For this review, take the finished solid that the model builds, in its own axes (mm). A direction names the side the tool comes from. Round coordinates to 2 decimals unless told otherwise and drop trailing zeros. Loops run counter-clockwise (first coordinate to the right, second up) from the corner with the lowest first, then second, coordinate; pieces in that order, holes last.
1. Clearance check with flat-ended pins moving along their axes: pin 1 Ø1 at (y, z) = (14.5, -11.5) entering from -X; pin 2 Ø2.5 at (x, z) = (10, -6) entering from -Y; pin 3 Ø5 at (x, z) = (10, -20) entering from +Y. State where each tip first meets the part, or that it passes through.
2. Consider section C-C on y = 48. State the section outline as (x, z) points, then the cut area to 3 significant figures.
3. Consider section D-D on z = -13. State the section outline as (x, y) points, then the cut area to 3 significant figures.
4. Tool access review of faces 4 (the flat face through (0, 1, -13)), 5 (the flat face through (41, 27, -1)), 6 (the flat face through (42, 38, -23)): name each direction out of +Z, -Z, +X, -X, +Y, -Y from which nothing blocks a thin tool from reaching the whole face with its end or side.
5. Draft analysis for pull direction Y (two halves, no side actions). For faces 1 (the flat face through (22, 0, -13)), 2 (the flat face through (42, 23, -26)), 3 (the cylindrical face through (42.479, 60.336, -18.325)), state which applies: released by +Y, released by -Y, zero draft, split by the parting line, or undercut.
6. Consider section A-A on y = 14.5. State the section outline as (x, z) points, then the cut area to 3 significant figures.
7. To check wall thickness, follow line 1 along Y through (x, z) = (43.2, -8); line 2 along X through (y, z) = (1, -13); line 3 along Y through (x, z) = (4, -2.5). State the ranges of each line that lie inside material, in increasing order.
8. Consider section B-B on x = 3. State the section outline as (y, z) points, then the cut area to 3 significant figures.
from build123d import *

# Parameters (mm, degrees)
CROQUIS1_R              = 1.5
CROQUIS1_R_2            = 1.58
SALIENTE_EXTRUIR1_DEPTH = 3
CROQUIS2_W              = 3
CROQUIS2_H              = 26
SALIENTE_EXTRUIR2_DEPTH = 15
CROQUIS3_R              = 1.5
CORTAR_EXTRUIR1_DEPTH   = 15
CROQUIS4_W              = 3
CROQUIS4_H              = 3
SALIENTE_EXTRUIR3_DEPTH = 40.3
CROQUIS5_W              = 3
CROQUIS5_H              = 26
SALIENTE_EXTRUIR5_DEPTH = 7.5
CROQUIS6_R              = 1.5
CORTAR_EXTRUIR2_DEPTH   = 7.5


with BuildPart() as part:
    # Croquis1 → Saliente-Extruir1 (new body)
    with BuildSketch(Plane(origin=(0, 0, 0), x_dir=(1, 0, 0), z_dir=(0, 1, 0))):
        with BuildLine():
            Line((0, 1.5), (0, 24.5))
            ThreePointArc((0, 24.5), (0.439339828, 25.560660172), (1.5, 26))
            Line((1.5, 26), (44, 26))
            Line((44, 26), (44, 0))
            Line((44, 0), (1.5, 0))
            ThreePointArc((1.5, 0), (0.439339828, 0.439339828), (0, 1.5))
        make_face()
        with Locations(Location((10, 13, 0), (0, 0, 270))):
            Circle(CROQUIS1_R, mode=Mode.SUBTRACT)
        with Locations(Location((17, 13, 0), (0, 0, 270))):
            Circle(CROQUIS1_R, mode=Mode.SUBTRACT)
        with Locations(Location((10, 20, 0), (0, 0, 270))):
            Circle(CROQUIS1_R, mode=Mode.SUBTRACT)
        with Locations(Location((10, 6, 0), (0, 0, 270))):
            Circle(CROQUIS1_R, mode=Mode.SUBTRACT)
        with Locations(Location((3, 13, 0), (0, 0, 270))):
            Circle(CROQUIS1_R_2, mode=Mode.SUBTRACT)
    extrude(amount=SALIENTE_EXTRUIR1_DEPTH)

    # Croquis2 → Saliente-Extruir2 (add)
    with BuildSketch(Plane(origin=(0, 3, 0), x_dir=(1, 0, 0), z_dir=(0, 1, 0))):
        with Locations((42.5, 13)):
            Rectangle(CROQUIS2_W, CROQUIS2_H)
    extrude(amount=SALIENTE_EXTRUIR2_DEPTH)

    # Croquis3 → Cortar-Extruir1 (cut)
    with BuildSketch(Plane.ZY.offset(-41)):
        with Locations((-18, 14.5)):
            Circle(CROQUIS3_R)
        with Locations((-8, 14.5)):
            Circle(CROQUIS3_R)
    extrude(amount=-CORTAR_EXTRUIR1_DEPTH, mode=Mode.SUBTRACT)

    # Croquis4 → Saliente-Extruir3 (add)
    with BuildSketch(Plane(origin=(0, 18, 0), x_dir=(1, 0, 0), z_dir=(0, 1, 0))):
        with Locations((42.5, 24.5)):
            Rectangle(CROQUIS4_W, CROQUIS4_H)
        with Locations((42.5, 1.5)):
            Rectangle(CROQUIS4_W, CROQUIS4_H)
    extrude(amount=SALIENTE_EXTRUIR3_DEPTH)

    # Croquis5 → Saliente-Extruir5 (add)
    with BuildSketch(Plane(origin=(0, 58.3, 0), x_dir=(1, 0, 0), z_dir=(0, 1, 0))):
        with Locations((42.5, 13)):
            Rectangle(CROQUIS5_W, CROQUIS5_H)
    extrude(amount=SALIENTE_EXTRUIR5_DEPTH)

    # Croquis6 → Cortar-Extruir2 (cut)
    with BuildSketch(Plane.ZY.offset(-41)):
        with Locations((-18, 61.8)):
            Circle(CROQUIS6_R)
        with Locations((-8, 61.8)):
            Circle(CROQUIS6_R)
    extrude(amount=-CORTAR_EXTRUIR2_DEPTH, mode=Mode.SUBTRACT)


solid = part.part
Resolved:
1. pin 1: stops at x = 41
1. pin 2: passes through
1. pin 3: stops at y = 3
2. outline: (41, -26) - (44, -26) - (44, -23) - (41, -23) - close; (41, -3) - (44, -3) - (44, 0) - (41, 0) - close
2. area: 18.0 mm2
3. outline: (0, 0) - (1.42, 0) - (1.42, 3) - (0, 3) - close; (4.58, 0) - (8.5, 0) - (8.5, 3) - (4.58, 3) - close; (11.5, 0) - (15.5, 0) - (15.5, 3) - (11.5, 3) - close; (18.5, 0) - (44, 0) - (44, 18) - (41, 18) - (41, 3) - (18.5, 3) - close; (41, 58.3) - (44, 58.3) - (44, 65.8) - (41, 65.8) - close
3. area: 172 mm2
4. face 4: +Z, -Z, -X, +Y, -Y
4. face 5: +Z, -Z, -X, +Y
4. face 6: +X, -X
5. face 1: released by -Y
5. face 2: zero draft
5. face 3: undercut
6. outline: (41, -26) - (44, -26) - (44, -19.5) - (41, -19.5) - close; (41, -16.5) - (44, -16.5) - (44, -9.5) - (41, -9.5) - close; (41, -6.5) - (44, -6.5) - (44, 0) - (41, 0) - close
6. area: 60.0 mm2
7. line 1: y = 0 to 13, 16 to 18, 58.3 to 60.3, 63.3 to 65.8
7. line 2: x = 0 to 1.42, 4.58 to 8.5, 11.5 to 15.5, 18.5 to 44
7. line 3: y = 0 to 3
8. outline: (0, -26) - (3, -26) - (3, -14.58) - (0, -14.58) - close; (0, -11.42) - (3, -11.42) - (3, 0) - (0, 0) - close
8. area: 68.5 mm2
